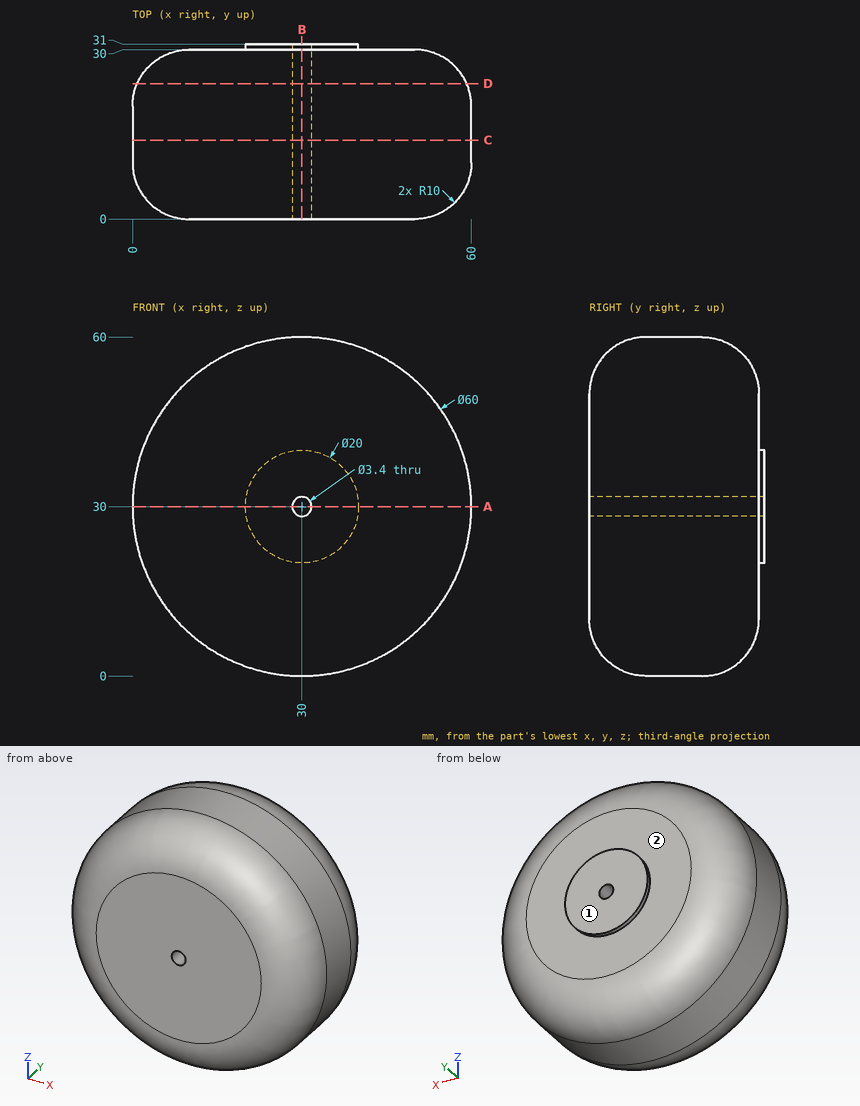
Could you check a few things on this drawing? It's one solid part, dimensions in mm from its lowest x, y, z. A direction names the side the tool comes from. Coordinates: 2 decimals unless noted, no trailing zeros. Write each loop counter-clockwise with the first axis right and the second up, starting at its lowest first coordinate (ties: lowest second). Pieces come first, ordered by that corner, then holes.
1) If we section it at C-C (y = 14): List the corners of the cut face in (x, z) for me.
Filled in:
outline: circle Ø60 at (30, 30); hole circle Ø3.4 at (30, 30)
2) Which directions (+Z, -Z, +X, -X, +Y, -Y) give clear straight access to the entire face, cutting with the end or side of a thin tool? Please do the marked faces 1 and 2.
Filled in:
face 1: +Z, -Z, +X, -X, +Y
face 2: +Y
3) If we section it at D-D (y = 24): List the corners of the cut face in (x, z) for me.
Filled in:
outline: circle Ø58.33 at (30, 30); hole circle Ø3.4 at (30, 30)
4) If we section it at A-A (z = 30): List the corners of the cut face in (x, y) for me.
Filled in:
outline: (0, 10) arc R10 ccw to (10, 0) - (28.3, 0) - (28.3, 31) - (20, 31) - (20, 30) - (10, 30) arc R10 ccw to (0, 20) - close; (31.7, 0) - (50, 0) arc R10 ccw to (60, 10) - (60, 20) arc R10 ccw to (50, 30) - (40, 30) - (40, 31) - (31.7, 31) - close
5) If I drill on line 1 (Z direction, x = 30, y = 13); line 2 (Y direction, x = 17.5, z = 40); line 3 (Z direction, x = 30, y = 23), over which ranges is the centre line in solid material (lowest first)?
Filled in:
line 1: z = 0 to 28.3, 31.7 to 60
line 2: y = 0 to 30
line 3: z = 0.46 to 28.3, 31.7 to 59.54
6) I'm going to push flat-ended pins straight in: pin 1 (4 mm diameter, centred on x = 21.5, y = 18, fed in from -Z); pin 2 (3 mm diameter, centred on x = 19, y = 7, fed in from -Z); pin 3 (2 mm diameter, centred on x = 52.5, z = 39.5, fed in from -Y). Where does each tip first touch, or does it pass through?
Filled in:
pin 1: stops at z = 0.71
pin 2: stops at z = 1.88
pin 3: stops at y = 0.6
7) If we section it at B-B (x = 30): List the corners of the cut face in (y, z) for me.
Filled in:
outline: (0, 10) arc R10 ccw to (10, 0) - (20, 0) arc R10 ccw to (30, 10) - (30, 20) - (31, 20) - (31, 28.3) - (0, 28.3) - close; (0, 31.7) - (31, 31.7) - (31, 40) - (30, 40) - (30, 50) arc R10 ccw to (20, 60) - (10, 60) arc R10 ccw to (0, 50) - close
